Build history of the part. All positions in model axes, mm. A direction names the side the tool comes from. Give positions to 0.01 mm unless a question says otherwise; leave off trailing zeros. Loops run counter-clockwise (first coordinate to the right, second up) from the corner with the lowest first, then second, coordinate; pieces in that order, holes last. Notation, with made-up numbers: (55, 45.5) -> (104, 45.5) arc R14 cw to (104, 52.5) -> close; hole circle Ø11 at (22.25, -16.75). An arc over 180 degrees is marked (long way). Answer as a JSON object with one key per item and string values. Group by question number.
Q1. Drop flat-ended pins along their axis: pin 1 (10 mm diameter, centred on x = -76.5, y = 3, fed in from -Z); pin 2 (8 mm diameter, centred on x = -30.31, y = -17.5, fed in from +Z); pin 3 (6 mm diameter, centred on y = 61, z = -88.5, fed in from +X). Give the stop position or say it passes through.
Q2. Two-plate mould, pull along X, no slides. Class faces 6 (the flat face through (55, -87, 50.8)), 7 (the cylindrical face through (28.7, -14.97, 9.86)), 8 (the cylindrical face through (-11.923, -53.692, 27.296)): pulls with the +X half, pulls with the -X half, needs draft (parallel to the pull), parting line crosses it, or undercut.
Q3. Wall check: probe 1 along X at (y, z) = (-80, -2.5); probe 2 along X at (y, z) = (-8, -116.5); probe 3 along Y at (x, z) = (-109, -69). Give the ranges that are in metal, low to high. Write a range as from..to.
Q4. Band-saw the part on B-B, the plane x = 0. Write the cut outline in (y, z), plus the area to 3 significant figures.
Q5. Band-saw the part on A-A, the plane z = -33. Write the cut outline in (x, y), plus the area to 3 significant figures.
Q6. Tool access for faces 1 (the flat face through (99, -99.707, -92)), 2 (the flat face through (-105, -56, -98)), 3 (the cylindrical face through (110.14, 37.79, -40.47)), 4 (the flat face through (41, -41, 34.8)), 5 (the flat face through (-109.86, 15.37, -107.126)): list every direction of +Z, -Z, +X, -X, +Y, -Y with a clear straight run to the whole face (end or side of a thin tool).
from build123d import *

# Parameters (mm, degrees)
SKETCH_1_R               = 100
SKETCH_1_R_2             = 95
EXTRUDE_1_DEPTH          = 50.8
SKETCH_2_R               = 95
SKETCH_2_R_2             = 55
EXTRUDE_2_DEPTH          = 34.8
SKETCH_4_R               = 55
SKETCH_4_R_2             = 3
SKETCH_4_R_3             = 27.5
EXTRUDE_3_DEPTH          = 20
SKETCH_5_R               = 3
CUT_EXTRUDE_2_DEPTH      = 20
PATTERN_CIRCULAR_3_COUNT = 6
EXTRUDE_4_DEPTH          = 50.8
SKETCH_7_W               = 80
SKETCH_7_H               = 200
EXTRUDE_5_DEPTH          = 100
SKETCH_8_W               = 80
SKETCH_8_H               = 200
CUT_EXTRUDE_3_DEPTH      = 100
CUT_EXTRUDE_5_DEPTH      = 218.118953572
CUT_EXTRUDE_5_DEPTH_BACK = 100
SKETCH_11_W              = 60
SKETCH_11_H              = 200
SKETCH_15_W              = 20
SKETCH_15_H              = 200
EXTRUDE_6_DEPTH          = 30
CUT_EXTRUDE_13_DEPTH     = 20
SKETCH_19_W              = 36
SKETCH_19_H              = 160
CUT_EXTRUDE_14_DEPTH     = 10
SKETCH_20_R              = 3
CUT_EXTRUDE_15_DEPTH     = 10
SKETCH_21_W              = 21.45
SKETCH_21_H              = 200
EXTRUDE_9_DEPTH          = 82.5
SKETCH_26_R              = 40
CUT_EXTRUDE_19_DEPTH     = 17.45
SKETCH_27_R              = 17.5
CUT_EXTRUDE_20_DEPTH     = 17.45
FILLET_1_R               = 1
FILLET_2_R               = 1
SKETCH_31_W              = 42.314213562
SKETCH_31_H              = 199.414213562
EXTRUDE_11_DEPTH         = 20
CUT_EXTRUDE_START        = -50
SKETCH_32_R              = 40
CUT_EXTRUDE_23_DEPTH     = 50
SKETCH_33_R              = 40
EXTRUDE_12_DEPTH         = 4
SKETCH_34_R              = 20
CUT_EXTRUDE_24_DEPTH     = 4
SKETCH_39_R              = 3
CUT_EXTRUDE_26_DEPTH     = 20


with BuildPart() as part:
    # 草图1 → 凸台-拉伸1 (new body)
    with BuildSketch(Plane.XY):
        Circle(SKETCH_1_R)
        Circle(SKETCH_1_R_2, mode=Mode.SUBTRACT)
    extrude(amount=EXTRUDE_1_DEPTH)

    # 草图2 → 凸台-拉伸2 (add)
    with BuildSketch(Plane.XY):
        Circle(SKETCH_2_R)
        Circle(SKETCH_2_R_2, mode=Mode.SUBTRACT)
    extrude(amount=EXTRUDE_2_DEPTH)

    # 草图4 → 凸台-拉伸3 (add)
    with BuildSketch(Plane.XY):
        Circle(SKETCH_4_R)
        with Locations((0, -35)):
            Circle(SKETCH_4_R_2, mode=Mode.SUBTRACT)
        Circle(SKETCH_4_R_3, mode=Mode.SUBTRACT)
    extrude(amount=EXTRUDE_3_DEPTH)

    # 草图5 → 切除-拉伸2 (cut)
    with BuildSketch(Plane(origin=(0, 0, 0), x_dir=(-1, 0, 0), z_dir=(0, 0, -1))):
        with Locations((0, 35)):
            Circle(SKETCH_5_R)
    cut_extrude_2 = extrude(amount=-CUT_EXTRUDE_2_DEPTH, mode=Mode.SUBTRACT)

    # 阵列(圆周)3: 切除-拉伸2 ×6 about axis
    pattern_circular_3_axis = Axis((0, 0, 0), (0, 0, 1))
    for i in range(1, PATTERN_CIRCULAR_3_COUNT):
        add(cut_extrude_2.rotate(pattern_circular_3_axis, i * 360 / PATTERN_CIRCULAR_3_COUNT), mode=Mode.SUBTRACT)

    # 草图6 → 凸台-拉伸4 (add)
    with BuildSketch(Plane(origin=(0, 0, 0), x_dir=(-1, 0, 0), z_dir=(0, 0, -1))):
        with BuildLine():
            ThreePointArc((100, 0), (70.71067814, -70.710678097), (6.1e-08, -100))
            Line((6.1e-08, -100), (200, -100))
            Line((200, -100), (200, 100))
            Line((200, 100), (0, 100))
            ThreePointArc((0, 100), (70.710678119, 70.710678119), (100, 0))
        make_face()
        with BuildLine():
            Line((-200, 100), (-200, -100))
            Line((-200, -100), (6.1e-08, -100))
            ThreePointArc((6.1e-08, -100), (-100, -3e-08), (0, 100))
            Line((0, 100), (-200, 100))
        make_face()
    extrude(amount=-EXTRUDE_4_DEPTH)

    # 草图7 → 凸台-拉伸5 (add)
    with BuildSketch(Plane(origin=(0, 0, 0), x_dir=(-1, 0, 0), z_dir=(0, 0, -1))):
        with Locations((80, 0)):
            Rectangle(SKETCH_7_W, SKETCH_7_H)
    extrude(amount=EXTRUDE_5_DEPTH)

    # 草图8 → 切除-拉伸3 (cut)
    with BuildSketch(Plane(origin=(0, 0, 0), x_dir=(-1, 0, 0), z_dir=(0, 0, -1))):
        with Locations((160, 0)):
            Rectangle(SKETCH_8_W, SKETCH_8_H)
    cut_extrude_3 = extrude(amount=-CUT_EXTRUDE_3_DEPTH, mode=Mode.SUBTRACT)

    # 镜向2: 切除-拉伸3 across plane
    add(cut_extrude_3.mirror(Plane(origin=(0, 0, 0), x_dir=(0, 0, 1), z_dir=(1, 0, 0))), mode=Mode.SUBTRACT)

    # 草图11 → 切除-拉伸5 (cut, two sides: drawn at the far end of the back side and taken through both)
    with BuildSketch(Plane(origin=(0, 0, -100), x_dir=(-1, 0, 0), z_dir=(0, 0, -1)).offset(-CUT_EXTRUDE_5_DEPTH_BACK)):
        with Locations((70, 0)):
            Rectangle(SKETCH_11_W, SKETCH_11_H)
    extrude(amount=CUT_EXTRUDE_5_DEPTH + CUT_EXTRUDE_5_DEPTH_BACK, mode=Mode.SUBTRACT)

    # 草图15 → 凸台-拉伸6 (add)
    with BuildSketch(Plane(origin=(0, 0, -100), x_dir=(-1, 0, 0), z_dir=(0, 0, -1))):
        with Locations((110, 0)):
            Rectangle(SKETCH_15_W, SKETCH_15_H)
    extrude(amount=EXTRUDE_6_DEPTH)

    # 草图16 → 切除-拉伸13 (cut)
    with BuildSketch(Plane(origin=(-100, 0, 0), x_dir=(0, 0, -1), z_dir=(1, 0, 0))):
        Polygon((80, 0), (44, 0), (62, -31.176914536), (80, -31.176914536), align=None)
        Polygon((62, 31.176914536), (44, 0), (80, 0), (80, 31.176914536), align=None)
        Polygon((80, 31.176914536), (80, 0), (116, 0), (98, 31.176914536), align=None)
        Polygon((116, 0), (80, 0), (80, -31.176914536), (98, -31.176914536), align=None)
    extrude(amount=-CUT_EXTRUDE_13_DEPTH, mode=Mode.SUBTRACT)

    # 草图19 → 切除-拉伸14 (cut)
    with BuildSketch(Plane(origin=(-100, 0, 0), x_dir=(0, 0, -1), z_dir=(1, 0, 0))):
        with Locations((80, 0)):
            Rectangle(SKETCH_19_W, SKETCH_19_H)
    extrude(amount=-CUT_EXTRUDE_14_DEPTH, mode=Mode.SUBTRACT)

    # 草图20 → 切除-拉伸15 (cut)
    with BuildSketch(Plane(origin=(-110, 0, 0), x_dir=(0, 0, -1), z_dir=(1, 0, 0))):
        with Locations(Location((80, 62, 0), (0, 0, 90))):
            Circle(SKETCH_20_R)
    cut_extrude_15 = extrude(amount=-CUT_EXTRUDE_15_DEPTH, mode=Mode.SUBTRACT)

    # 镜向6: 切除-拉伸15 across plane
    add(cut_extrude_15.mirror(Plane.ZX), mode=Mode.SUBTRACT)

    # 草图21 → 凸台-拉伸9 (add)
    with BuildSketch(Plane(origin=(0, 0, 0), x_dir=(-1, 0, 0), z_dir=(0, 0, -1))):
        with Locations((-109.275, 0)):
            Rectangle(SKETCH_21_W, SKETCH_21_H)
    extrude_9 = extrude(amount=EXTRUDE_9_DEPTH)

    # 草图26 → 切除-拉伸19 (cut)
    with BuildSketch(Plane.ZY.offset(-98.55)):
        with Locations((-82.5, 0)):
            Circle(SKETCH_26_R)
    cut_extrude_19 = extrude(amount=-CUT_EXTRUDE_19_DEPTH, mode=Mode.SUBTRACT)

    # 草图27 → 切除-拉伸20 (cut)
    with BuildSketch(Plane.ZY.offset(-116)):
        with Locations((-82.5, 0)):
            Circle(SKETCH_27_R)
    cut_extrude_20 = extrude(amount=-CUT_EXTRUDE_20_DEPTH, mode=Mode.SUBTRACT)

    # 镜向8: 凸台-拉伸9, 切除-拉伸19, 切除-拉伸20 across plane
    add(extrude_9.mirror(Plane(origin=(98.55, 0, 0), x_dir=(0, 0, 1), z_dir=(1, 0, 0))))
    add(cut_extrude_19.mirror(Plane(origin=(98.55, 0, 0), x_dir=(0, 0, 1), z_dir=(1, 0, 0))), mode=Mode.SUBTRACT)
    add(cut_extrude_20.mirror(Plane(origin=(98.55, 0, 0), x_dir=(0, 0, 1), z_dir=(1, 0, 0))), mode=Mode.SUBTRACT)

    # 圆角1
    fillet_1_edges = [part.edges().sort_by_distance(p)[0] for p in [
        (120, 100, -15.85),
        (120, -100, -15.85),
        (98.55, -100, -82.5),
        (98.55, 100, -82.5),
        (120, 58.75, -82.5),
        (116, -28.75, -82.5),
        (98.55, 40, -82.5),
        (98.55, -40, -82.5),
        (116, 28.75, -82.5),
        (116, 0, -65),
        (120, -58.75, -82.5),
        (120, 0, -65),
        (118, -17.5, -82.5),
        (118, 17.5, -82.5),
        (77.1, 58.75, -82.5),
        (77.1, -100, -41.25),
        (77.1, 100, -41.25),
        (81.1, 28.75, -82.5),
        (81.1, 0, -42.5),
        (81.1, -28.75, -82.5),
        (81.1, 0, -65),
        (77.1, -58.75, -82.5),
        (79.1, 17.5, -82.5),
        (77.1, 0, -65),
        (79.1, -17.5, -82.5),
    ]]
    fillet(fillet_1_edges, radius=FILLET_1_R)

    # 圆角2
    fillet_2_edges = [part.edges().sort_by_distance(p)[0] for p in [
        (119.707106781, -99.707106781, 50.8),
        (119.707106781, 99.707106781, 50.8),
        (-120, 0, 50.8),
        (-0.5, -100, 50.8),
        (-0.5, 100, 50.8),
        (120, 0, 50.8),
        (-10.95, -100, 0),
        (-10.95, 100, 0),
        (-100, -100, -65),
        (-120, -100, -39.6),
        (-110, -100, -130),
        (-100, 100, -65),
        (-100, 0, -130),
        (-110, 100, -130),
        (-120, 0, -130),
        (-120, 100, -39.6),
    ]]
    fillet(fillet_2_edges, radius=FILLET_2_R)

    # 草图31 → 凸台-拉伸11 (add)
    with BuildSketch(Plane(origin=(0, 0, -82.5), x_dir=(-1, 0, 0), z_dir=(0, 0, -1))):
        with Locations((-98.55, 0)):
            Rectangle(SKETCH_31_W, SKETCH_31_H)
    extrude(amount=EXTRUDE_11_DEPTH)

    # 草图32 → 切除-拉伸23 (cut)
    with BuildSketch(Plane(origin=(120, 0, 0), x_dir=(0, 0, -1), z_dir=(1, 0, 0)).offset(CUT_EXTRUDE_START)):
        with Locations((82.5, 0)):
            Circle(SKETCH_32_R)
    extrude(amount=CUT_EXTRUDE_23_DEPTH, mode=Mode.SUBTRACT)

    # 草图33 → 凸台-拉伸12 (add)
    with BuildSketch(Plane.ZY.offset(-77.392893219)):
        with Locations((-82.5, 0)):
            Circle(SKETCH_33_R)
    extrude(amount=-EXTRUDE_12_DEPTH)

    # 草图34 → 切除-拉伸24 (cut)
    with BuildSketch(Plane.ZY.offset(-77.392893219)):
        with Locations((-82.5, 0)):
            Circle(SKETCH_34_R)
    extrude(amount=-CUT_EXTRUDE_24_DEPTH, mode=Mode.SUBTRACT)

    # 草图39 → 切除-拉伸26 (cut)
    with BuildSketch(Plane(origin=(120, 0, 0), x_dir=(0, 0, -1), z_dir=(1, 0, 0))):
        with Locations(Location((42.5, 40, 0), (0, 0, 90))):
            Circle(SKETCH_39_R)
        with Locations(Location((42.5, -40, 0), (0, 0, 90))):
            Circle(SKETCH_39_R)
    extrude(amount=-CUT_EXTRUDE_26_DEPTH, mode=Mode.SUBTRACT)


solid = part.part
Worked answers:
{
 "1": {"pin 1": "z = 0", "pin 2": "z = 20", "pin 3": "x = 119.71"},
 "2": {"face 6": "needs draft", "face 7": "undercut", "face 8": "undercut"},
 "3": {"probe 1": "-120..-100, 77.1..120", "probe 2": "-120..-100, 77.39..81.39", "probe 3": "-100..-80, 80..100"},
 "4": {"outline": "(-100, 1) arc R1 ccw to (-99, 0) -> (-38, 0) -> (-38, 20) -> (-55, 20) -> (-55, 34.8) -> (-95, 34.8) -> (-95, 50.8) -> (-99, 50.8) arc R1 ccw to (-100, 49.8) -> close; (-32, 0) -> (-27.5, 0) -> (-27.5, 20) -> (-32, 20) -> close; (27.5, 0) -> (32, 0) -> (32, 20) -> (27.5, 20) -> close; (38, 0) -> (99, 0) arc R1 ccw to (100, 1) -> (100, 49.8) arc R1 ccw to (99, 50.8) -> (95, 50.8) -> (95, 34.8) -> (55, 34.8) -> (55, 20) -> (38, 20) -> close", "area": "4,150 mm2"},
 "5": {"outline": "(-120, -99) arc R1 ccw to (-119, -100) -> (-101, -100) arc R1 ccw to (-100, -99) -> (-100, 99) arc R1 ccw to (-101, 100) -> (-119, 100) arc R1 ccw to (-120, 99) -> close; (77.1, -99) arc R1 ccw to (78.1, -100) -> (119, -100) arc R1 ccw to (120, -99) -> (120, 99) arc R1 ccw to (119, 100) -> (78.1, 100) arc R1 ccw to (77.1, 99) -> close", "area": "12,600 mm2"},
 "6": {"face 1": "-Z, +X, -Y", "face 2": "none", "face 3": "+X", "face 4": "+Z", "face 5": "-X"}
}
